Check sheet for the modelled part. Datum: model origin and axes. Units: mm. A direction names the side the tool comes from. Give positions to 0.01 mm unless a question says otherwise; leave off trailing zeros. Write each loop counter-clockwise with the first axis right and the second up, starting at its lowest first coordinate (ties: lowest second). Pieces come first, ordered by that corner, then holes.
from build123d import *

# Parameters (mm, degrees)
SWEEP_1_PROFILE_R   = 18
SKETCH_35_R         = 18
EXTRUDE_1_DEPTH     = 85.4
SWEEP_1_2_PROFILE_R = 13.6
SKETCH_56_R         = 13.6
CUT_EXTRUDE_3_DEPTH = 103.698548903
SKETCH_33_R         = 16
CUT_EXTRUDE_1_DEPTH = 22.2
SKETCH_34_R         = 16
CUT_EXTRUDE_2_DEPTH = 22.2
CUT_EXTRUDE_START   = -22.2
SKETCH_56_4_R       = 16
CUT_EXTRUDE_4_DEPTH = 22.2


with BuildPart() as part:
    # Sweep 1: sweep along a path in Sketch 1
    with BuildLine(Plane(origin=(0, 0, 0), x_dir=(1, 0, 0), z_dir=(0, 1, 0))) as sweep_1_path:
        Line((-41.4, 41.4), (0, 0))
        Line((0, 0), (30, 0))
    # Sweep 1 profile (on start of the path) → Sweep 1 (sweep)
    with BuildSketch(Plane(origin=(-41.4, 0, -41.4), x_dir=(0.7071067811865488, 0, -0.7071067811865462), z_dir=(0.7071067811865462, 0, 0.7071067811865488))):
        Circle(SWEEP_1_PROFILE_R)
    sweep(path=sweep_1_path.line, transition=Transition.RIGHT)

    # Sketch 35 → Extrude 1 (add)
    with BuildSketch(Plane(origin=(30, 0, 0), x_dir=(0, 0, -1), z_dir=(1, 0, 0))):
        Circle(SKETCH_35_R)
    extrude(amount=-EXTRUDE_1_DEPTH)

    # Sweep 1 2: sweep along a path in Sketch 1_11
    with BuildLine(Plane(origin=(0, 0, 0), x_dir=(1, 0, 0), z_dir=(0, 1, 0))) as sweep_1_2_path:
        Line((-41.4, 41.4), (0, 0))
        Line((0, 0), (30, 0))
    # Sweep 1 2 profile (on start of the path) → Sweep 1 2 (sweep, cut)
    with BuildSketch(Plane(origin=(-41.4, 0, -41.4), x_dir=(0.7071067811865488, 0, -0.7071067811865462), z_dir=(0.7071067811865462, 0, 0.7071067811865488))):
        Circle(SWEEP_1_2_PROFILE_R)
    sweep(path=sweep_1_2_path.line, transition=Transition.RIGHT, mode=Mode.SUBTRACT)

    # Sketch 56 → Cut-Extrude 3 (cut, through all)
    with BuildSketch(Plane.ZY.offset(55.4)):
        Circle(SKETCH_56_R)
    extrude(amount=-CUT_EXTRUDE_3_DEPTH, mode=Mode.SUBTRACT)

    # Sketch 33 → Cut-Extrude 1 (cut)
    with BuildSketch(Plane(origin=(30, 0, 0), x_dir=(0, 0, -1), z_dir=(1, 0, 0))):
        Circle(SKETCH_33_R)
    extrude(amount=-CUT_EXTRUDE_1_DEPTH, mode=Mode.SUBTRACT)

    # Sketch 34 → Cut-Extrude 2 (cut)
    with BuildSketch(Plane(origin=(-41.4, 0, -41.4), x_dir=(-0.7071067811865486, 0, 0.7071067811865465), z_dir=(-0.7071067811865465, 0, -0.7071067811865486))):
        Circle(SKETCH_34_R)
    extrude(amount=-CUT_EXTRUDE_2_DEPTH, mode=Mode.SUBTRACT)

    # Sketch 56_4 → Cut-Extrude 4 (cut)
    with BuildSketch(Plane.ZY.offset(55.4).offset(CUT_EXTRUDE_START)):
        with Locations(Location((0, 0, 0), (0, 0, 180))):
            Circle(SKETCH_56_4_R)
    extrude(amount=CUT_EXTRUDE_4_DEPTH, mode=Mode.SUBTRACT)


solid = part.part
1) Sectioned sample at A-A on y = 9.5. Record the boundary of the cut face in (x, z), then the cut area to 3 significant figures.
2) Scan lines: L1, parallel to Y at x = -22.5, z = 0; L2, parallel to Y at x = 19, z = 0; L3, parallel to X at y = 6, z = -17.5. Record each from-to range of solid material in increasing order.
3) Sectioned sample at C-C on y = 0. Give the number of separate pieces and of enclosed holes in the cut face, then the cut area to 3 significant figures.
4) Gauge pin test, flat ends, axial feed: pin 1 (5 mm diameter, centred on x = -33.5, y = -10.5, fed in from -Z); pin 2 (4 mm diameter, centred on y = 6.5, z = -11, fed in from +X); pin 3 (6 mm diameter, centred on x = -33, y = 1.5, fed in from -Z). Record the tip position at first contact, or that the pin passes through.
5) Draft check along Z on faces 5 (the flat face through (-52.8, -1.2, -30)), 6 (the flat face through (-33.2, -11, 9)), 7 (the flat face through (7.8, -12, 7)), 8 (the flat face through (30, 11, -12)). Enter one of: +Z half, -Z half, draft (parallel to the pull), parting line (faces both ways), or undercut.
6) Sectioned sample at B-B on z = 8.5. Record the boundary of the cut face in (x, y), then the cut area to 3 significant figures.
7) Access from +Z, -Z, +X, -X, +Y, -Y to the whole of each face (thin tool, end or side, straight path). Record for faces 1 (the cylindrical face through (-12.102, 0.791, 17.983)), 2 (the flat face through (-55.4, -11, 12)), 3 (the cylindrical face through (-44.145, 9.736, 12.697)), 4 (the cylindrical face through (19.06, -15.62, 3.47)).
Answers below:
1. outline: (-55.4, -15.29) - (-36.91, -15.29) - (-52.21, -30.59) - (-50.5, -32.3) - (-34.81, -16.6) - (-32.58, -18.82) - (-23.49, -9.73) - (-33.2, -9.73) - (-33.2, -12.87) - (-55.4, -12.87) - close; (-55.4, 12.87) - (-33.2, 12.87) - (-33.2, 9.73) - (7.8, 9.73) - (7.8, 12.87) - (30, 12.87) - (30, 15.29) - (-55.4, 15.29) - close; (-32.3, -50.5) - (-30.59, -52.21) - (6.33, -15.29) - (30, -15.29) - (30, -12.87) - (7.8, -12.87) - (7.8, -9.73) - (4.03, -9.73) - (-18.82, -32.58) - (-16.6, -34.81) - close
1. area: 788 mm2
2. L1: y = -18 to -13.6, 13.6 to 18
2. L2: y = -18 to -16, 16 to 18
2. L3: x = -41.5 to -38.48, -0.24 to 6.5
3. separate pieces: 5
3. enclosed holes: 0
3. area: 558 mm2
4. pin 1: stops at z = -51.8
4. pin 2: stops at x = 7.8
4. pin 3: stops at z = -52.8
5. face 5: -Z half
5. face 6: undercut
5. face 7: undercut
5. face 8: draft
6. outline: (-55.4, -15.87) - (30, -15.87) - (30, -13.56) - (7.8, -13.56) - (7.8, -10.62) - (-33.2, -10.62) - (-33.2, -13.56) - (-55.4, -13.56) - close; (-55.4, 13.56) - (-33.2, 13.56) - (-33.2, 10.62) - (7.8, 10.62) - (7.8, 13.56) - (30, 13.56) - (30, 15.87) - (-55.4, 15.87) - close
6. area: 636 mm2
7. face 1: none
7. face 2: +Z, -Z, -X, +Y, -Y
7. face 3: -X
7. face 4: +X
